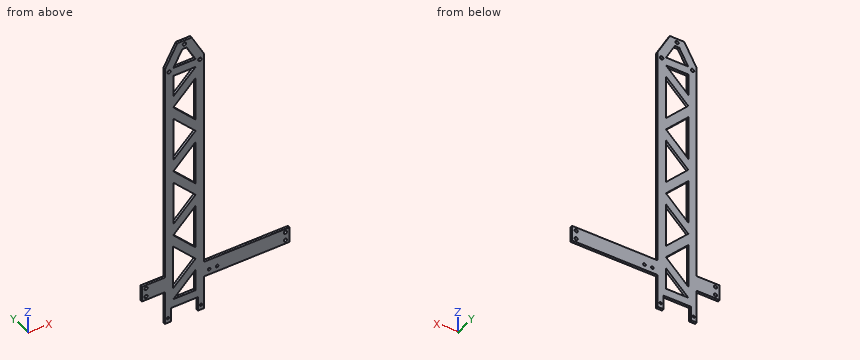
from build123d import *

# Parameters (mm, degrees)
SKETCH1_R           = 1.44
SKETCH1_R_2         = 1.35
SKETCH1_R_3         = 1
SKETCH1_R_4         = 1.125
BOSS_EXTRUDE1_DEPTH = 2


with BuildPart() as part:
    # Sketch1 → Boss-Extrude1 (new body)
    with BuildSketch(Plane(origin=(0, 0, 0), x_dir=(1, 0, 0), z_dir=(0, 1, 0))):
        Polygon((-17.332807681, 117.69771489), (-17.332807681, -38.346866508), (-6.997005855, -57.284094596), (4.918028523, -57.284094596), (15.167192319, -38.486712582), (15.167192319, 146.492065716), (86.167192319, 146.492065716), (86.167192319, 159.492065716), (15.167192319, 159.492065716), (15.167192319, 187.692065716), (10.237192319, 187.692065716), (10.237192319, 175.692065716), (-12.402807681, 175.692065716), (-12.402807681, 187.692065716), (-17.332807681, 187.692065716), (-17.332807681, 159.492065716), (-36.332807681, 159.492065716), (-36.332807681, 146.492065716), (-17.332807681, 146.492065716), align=None)
        with Locations((-13.842807681, -34.799722329)):
            Circle(SKETCH1_R, mode=Mode.SUBTRACT)
        with Locations((-1.042807681, -54.059722329)):
            Circle(SKETCH1_R, mode=Mode.SUBTRACT)
        Polygon((-2.842807681, -50.284094596), (-10.225590468, -36.757379986), (8.137192319, -36.757379986), (0.761829434, -50.284094596), align=None, mode=Mode.SUBTRACT)
        with Locations((11.757192319, -34.799722329)):
            Circle(SKETCH1_R, mode=Mode.SUBTRACT)
        Polygon((8.167192319, -29.757379986), (-10.332807681, -29.757379986), (-10.332807681, -11.546628322), align=None, mode=Mode.SUBTRACT)
        Polygon((8.167192319, -19.934969699), (-10.332807681, -1.724218034), (8.167192319, 17.069624543), align=None, mode=Mode.SUBTRACT)
        Polygon((8.167192319, 27.048047931), (-10.332807681, 8.254205353), (-10.332807681, 45.258799595), align=None, mode=Mode.SUBTRACT)
        Polygon((8.167192319, 36.870458218), (-10.332807681, 55.081209882), (8.167192319, 73.87505246), align=None, mode=Mode.SUBTRACT)
        Polygon((8.167192319, 83.853475847), (-10.332807681, 65.05963327), (-10.332807681, 102.064227512), align=None, mode=Mode.SUBTRACT)
        Polygon((8.167192319, 93.675886135), (-10.332807681, 111.886637799), (8.167192319, 130.680480377), align=None, mode=Mode.SUBTRACT)
        with Locations((-32.832807681, 149.492065716)):
            Circle(SKETCH1_R_2, mode=Mode.SUBTRACT)
        with Locations((-32.832807681, 156.492065716)):
            Circle(SKETCH1_R_2, mode=Mode.SUBTRACT)
        with Locations((-14.867807681, 183.496000094)):
            Circle(SKETCH1_R_3, mode=Mode.SUBTRACT)
        Polygon((8.167192319, 140.658903764), (-10.361742255, 121.835667033), (-10.361742255, 158.89813761), align=None, mode=Mode.SUBTRACT)
        with Locations((19.467192319, 154.892065716)):
            Circle(SKETCH1_R_4, mode=Mode.SUBTRACT)
        Polygon((8.167192319, 150.481314052), (-10.332807681, 168.692065716), (8.167192319, 168.692065716), align=None, mode=Mode.SUBTRACT)
        with Locations((12.702192319, 183.496000094)):
            Circle(SKETCH1_R_3, mode=Mode.SUBTRACT)
        with Locations((26.031178731, 154.892065716)):
            Circle(SKETCH1_R_4, mode=Mode.SUBTRACT)
        with Locations((82.667192319, 149.492065716)):
            Circle(SKETCH1_R_2, mode=Mode.SUBTRACT)
        with Locations((82.667192319, 156.492065716)):
            Circle(SKETCH1_R_2, mode=Mode.SUBTRACT)
    extrude(amount=BOSS_EXTRUDE1_DEPTH)


solid = part.part
Verification items for the finished model (mm, model axes). Round coordinates to 2 decimals unless told otherwise and drop trailing zeros. Order: outer loops, then holes, each group sorted by start corner. A loop starts at its lowest first (then second) coordinate and runs counter-clockwise, first axis right, second up. Notation, with made-up numbers: (-20.75, 35.5) -> (25.25, 35.5) arc R14 cw to (25.25, 58.5) -> close; hole circle Ø9 at (73.5, -37). An arc over 180 degrees is marked (long way). Put each result on its own line as item: value.
1) Section check C-C (x = 49). Record the cut outline in (y, z).
Final values:
outline: (0, -159.49) -> (2, -159.49) -> (2, -146.49) -> (0, -146.49) -> close
2) Section check D-D (y = 1). Give the number of separate pieces and of enclosed holes in the cut face, then the cut area to 3 significant figures.
Final values:
separate pieces: 1
enclosed holes: 20
area: 6,070 mm^2
3) Section check B-B (z = -78). Record the cut outline in (x, y).
Final values:
outline: (-17.33, 0) -> (-10.33, 0) -> (-10.33, 2) -> (-17.33, 2) -> close; (2.41, 0) -> (15.17, 0) -> (15.17, 2) -> (2.41, 2) -> close
4) Depth check by flat-ended pin: pin 1 (0.6 mm diameter, centred on y = 1, z = -29, fed in from +X); pin 2 (0.6 mm diameter, centred on x = 4.5, y = 1.5, fed in from -Z); pin 3 (1 mm diameter, centred on y = 0.5, z = -140, fed in from -X). Enter the tip coordinate at first touch or a pass-through.
Final values:
pin 1: stops at x = 15.17
pin 2: stops at z = -175.69
pin 3: stops at x = -17.33
5) Section check A-A (z = -4). Record the cut outline in (x, y).
Final values:
outline: (-17.33, 0) -> (-4.7, 0) -> (-4.7, 2) -> (-17.33, 2) -> close; (8.17, 0) -> (15.17, 0) -> (15.17, 2) -> (8.17, 2) -> close
6) Material ranges on line 1 (X direction, y = 0.45, z = 33.5); line 2 (Z direction, x = 76.5, y = 1.25); line 3 (X direction, y = 1.3, z = 6), recorded low to high.
Final values:
line 1: x = -17.33 to -14.46, -13.22 to 11.14, 12.38 to 15.17
line 2: z = -159.49 to -146.49
line 3: x = -17.33 to -5.99, 8.17 to 15.17
